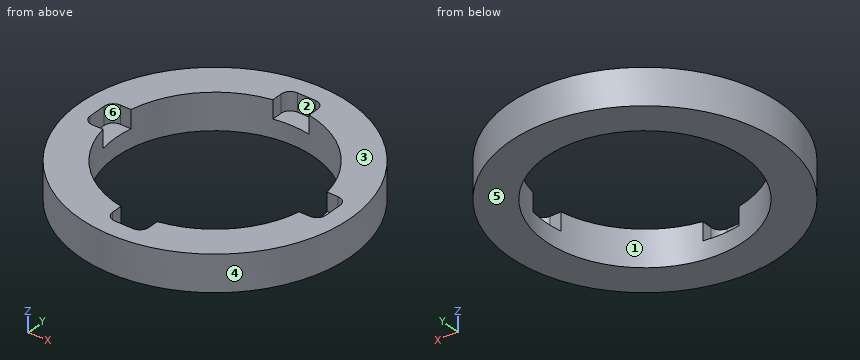
```python
from build123d import *

# Parameters (mm, degrees)
SKETCH1_R                = 47.5869
SKETCH1_R_2              = 34.8996
BOSS_EXTRUDE1_DEPTH      = 12.7
SKETCH2_W                = 12.7
SKETCH2_H                = 82.4992
CUT_EXTRUDE1_DEPTH       = 6.35
FILLET1_R                = 3.175
CIRPATTERN1_COUNT        = 2
CIRPATTERN1_ANGLE        = 90
FILLET1_OF_CIRPATTERN1_R = 3.175


with BuildPart() as part:
    # Sketch1 → Boss-Extrude1 (new body)
    with BuildSketch(Plane.XY):
        Circle(SKETCH1_R)
        Circle(SKETCH1_R_2, mode=Mode.SUBTRACT)
    extrude(amount=BOSS_EXTRUDE1_DEPTH)

    # Sketch2 → Cut-Extrude1 (cut)
    with BuildSketch(Plane.XY.offset(12.7)):
        Rectangle(SKETCH2_W, SKETCH2_H)
    cut_extrude1 = extrude(amount=-CUT_EXTRUDE1_DEPTH, mode=Mode.SUBTRACT)

    # Fillet1
    fillet1_edges = [part.edges().sort_by_distance(p)[0] for p in [
        (6.35, 41.2496, 9.525),
        (6.35, -41.2496, 9.525),
        (-6.35, -41.2496, 9.525),
        (-6.35, 41.2496, 9.525),
    ]]
    fillet(fillet1_edges, radius=FILLET1_R)

    # CirPattern1: Cut-Extrude1 ×2 about axis
    cirpattern1_axis = Axis((0, 0, 0), (0, 0, -1))
    for i in range(1, CIRPATTERN1_COUNT):
        add(cut_extrude1.rotate(cirpattern1_axis, i * CIRPATTERN1_ANGLE / (CIRPATTERN1_COUNT - 1)), mode=Mode.SUBTRACT)

    # Fillet1 of CirPattern1
    fillet1_of_cirpattern1_edges = [part.edges().sort_by_distance(p)[0] for p in [
        (41.2496, -6.35, 9.525),
        (-41.2496, -6.35, 9.525),
        (-41.2496, 6.35, 9.525),
        (41.2496, 6.35, 9.525),
    ]]
    fillet(fillet1_of_cirpattern1_edges, radius=FILLET1_OF_CIRPATTERN1_R)


solid = part.part
```
Design review of the part built by this model. Coordinates are the model's own, in mm. Face numbers are marked on the shaded views. A direction names the side the tool comes from. Coordinates: 2 decimals unless noted, no trailing zeros. Order: outer loops, then holes, each group sorted by start corner. A loop starts at its lowest first (then second) coordinate and runs counter-clockwise, first axis right, second up. Notation, with made-up numbers: (68, 19) - (91, 19) arc R19 cw to (91, 55) - close; hole circle Ø8 at (-9.75, 46). An arc over 180 degrees is marked (long way). One line per question, with ' | ' between items.
Q1. Consider section D-D, the plane x = -10.5. Give the boundary of the cut face in (y, z).
Answer key:
outline: (-46.41, 0) - (-33.28, 0) - (-33.28, 12.7) - (-46.41, 12.7) - close; (33.28, 0) - (46.41, 0) - (46.41, 12.7) - (33.28, 12.7) - close
Q2. Consider section A-A, the plane x = 0. Give the boundary of the cut face in (y, z).
Answer key:
outline: (-47.59, 0) - (-34.9, 0) - (-34.9, 6.35) - (-41.25, 6.35) - (-41.25, 12.7) - (-47.59, 12.7) - close; (34.9, 0) - (47.59, 0) - (47.59, 12.7) - (41.25, 12.7) - (41.25, 6.35) - (34.9, 6.35) - close
Q3. For the marked faces 5 and 6, list the 3-axis set-ups (+Z, -Z, +X, -X, +Y, -Y) from which the entire face can be reached by the end or side of a thin tool; tool diameter is ignored.
Answer key:
face 5: -Z, +X, -X, +Y, -Y | face 6: +Z
Q4. The part is to be moulded in two halves that separate along X. For the marked faces 1, 2, 3 and 4, say which applies: +X half, -X half, draft (parallel to the pull), parting line (faces both ways), or undercut.
Answer key:
face 1: undercut | face 2: undercut | face 3: draft | face 4: parting line
Q5. Clearance check with flat-ended pins moving along their axes: pin 1 Ø4 at (x, z) = (35.5, 8.5) entering from -Y; pin 2 Ø1.1 at (y, z) = (36, 9) entering from +X; pin 3 Ø1.1 at (y, z) = (37, 10.5) entering from -X; pin 4 Ø10 at (x, y) = (-1.5, 27.5) entering from +Z. State where each tip first meets the part, or that it passes through.
Answer key:
pin 1: stops at y = -33.8 | pin 2: stops at x = 31.75 | pin 3: stops at x = -30.59 | pin 4: passes through
Q6. To check wall thickness, follow line 1 along Y through (x, z) = (0, 7.5); line 2 along Y through (x, z) = (-1, 4); line 3 along X through (y, z) = (-24.5, 3.5). State the ranges of each line that lie inside material, in increasing order.
Answer key:
line 1: y = -47.59 to -41.25, 41.25 to 47.59 | line 2: y = -47.58 to -34.89, 34.89 to 47.58 | line 3: x = -40.8 to -24.85, 24.85 to 40.8
Q7. Consider section B-B, the plane z = 8.5. Give the boundary of the cut face in (x, y) (3 decimals), then the cut area to 3 significant figures.
Answer key:
outline: circle Ø95.174 at (0, 0); hole (-41.25, -3.175) arc R3.175 ccw to (-38.075, -6.35) - (-34.317, -6.35) arc R34.9 ccw to (-6.35, -34.317) - (-6.35, -38.075) arc R3.175 ccw to (-3.175, -41.25) - (3.175, -41.25) arc R3.175 ccw to (6.35, -38.075) - (6.35, -34.317) arc R34.9 ccw to (34.317, -6.35) - (38.075, -6.35) arc R3.175 ccw to (41.25, -3.175) - (41.25, 3.175) arc R3.175 ccw to (38.075, 6.35) - (34.317, 6.35) arc R34.9 ccw to (6.35, 34.317) - (6.35, 38.075) arc R3.175 ccw to (3.175, 41.25) - (-3.175, 41.25) arc R3.175 ccw to (-6.35, 38.075) - (-6.35, 34.317) arc R34.9 ccw to (-34.317, 6.35) - (-38.075, 6.35) arc R3.175 ccw to (-41.25, 3.175) - close | area: 2,970 mm2
